Autodesk Inventor part; units mm, degrees
ref_plane "YZ Plane" through (0, 0, 0) normal (1, 0, 0) x (0, 1, 0)
ref_plane "XZ Plane" through (0, 0, 0) normal (0, 1, 0) x (-1, 0, 0)
ref_plane "XY Plane" through (0, 0, 0) normal (0, 0, 1) x (1, 0, 0)
sketch "Sketch1" plane through (0, 0, 0) normal (0, 1, 0) x (-1, 0, 0)
  line L0 (900, 40) -> (-900, 40)
  line L1 (-900, 40) -> (-900, -40)
  line L2 (-900, -40) -> (900, -40)
  line L3 (900, -40) -> (900, 40)
  line L4 (900, 40) -> (-900, -40) construction
  line L5 (674.96, 40) -> (721.148, -40)
  line L6 (0, 40) -> (0, -40) construction
  line L7 (-674.96, 40) -> (-721.148, -40)
  point P0 (0, 0)
  point P1 (0, 0)
  dimension "d0" = 80
  dimension "d1" = 1800
  dimension "d3" = 120
  dimension "d6" = 674.96
  dimension "d7" = 120
  dimension "d8" = 674.96
extrude "Plate1" add sketch "Sketch1" along normal mid plane 3 contours L5 L2 L7 L0
sketch "Sketch2" plane through (0, -1.5, 0) normal (0, -1, 0) x (1, 0, 0)
  line L0 (-1.6, 40) -> (1.6, 40)
  line L1 (1.6, 40) -> (1.6, -1)
  line L2 (1.6, -1) -> (-1.6, -1)
  line L3 (-1.6, -1) -> (-1.6, 40)
  line L4 (-674.96, 40) -> (674.96, 40)
  point P0 (0, 0)
  point P1 (0, 40)
  dimension "d9" = 3.2
  dimension "d10" = 41
extrude "Extrusion1" cut sketch "Sketch2" against normal through all
pattern_linear "Rectangular Pattern1" count 5 spacing 240 along (1, 0, 0) of "Extrusion1" first direction both ways yes
equation "\"d7\" = d3"
equation "\"d8\" = d6"
equation "\"d2\" = Thickness"
equation "\"BendReliefWidth\" = Thickness"
equation "\"BendReliefDepth\" = 0.5 * Thickness"
equation "\"CornerReliefSize\" = 4 * Thickness"
equation "\"MinimumRemnant\" = 2 * Thickness"
equation "\"TransitionRadius\" = BendRadius"
equation "\"JacobiRadiusSize\" = BendRadius"
equation "\"GapSize\" = Thickness"
properties part number "MSC 203 GRID" material "Stainless Steel"
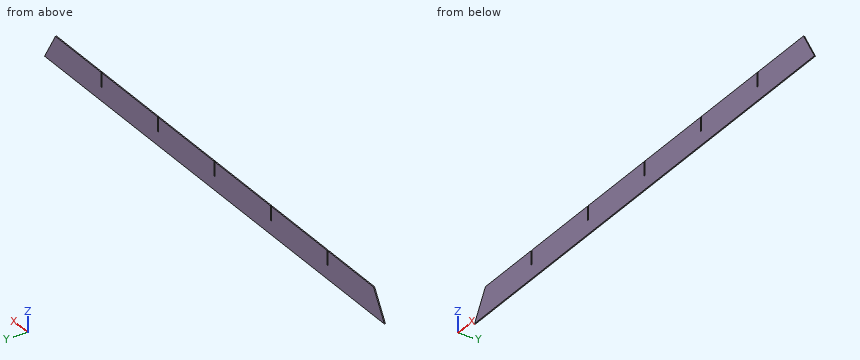
Check sheet for the modelled part. Datum: model origin and axes. Units: mm. Round coordinates to 2 decimals unless told otherwise and drop trailing zeros. Write each loop counter-clockwise with the first axis right and the second up, starting at its lowest first coordinate (ties: lowest second). Pieces come first, ordered by that corner, then holes. Notation, with made-up numbers: (-30.75, -2.75) -> (-20.75, -2.75) arc R20 cw to (-20.75, 34.25) -> close; hole circle Ø11 at (49.25, -6). An arc over 180 degrees is marked (long way). One line per question, with ' | ' between items. Start each with the question number.
1. Sectioned sample at B-B, the plane z = 25.5. Record the cut outline in (x, y), then the cut area to 3 significant figures.
2. Sectioned sample at A-A, the plane y = 0.3. Record the cut outline in (x, z), then the cut area to 3 significant figures.
3. Depth check by flat-ended pin: pin 1 (0.9 mm diameter, centred on x = 0, y = 0, fed in from +Z); pin 2 (1.5 mm diameter, centred on y = 0.5, z = 25.5, fed in from +X); pin 3 (0.9 mm diameter, centred on y = 0, z = 23.5, fed in from +X). Enter the tip coordinate at first touch or a pass-through.
4. Scan lines: line 1 along X through (y, z) = (0.1, 20); line 2 along X through (y, z) = (-1.3, 24); line 3 along X through (y, z) = (0.35, -32). Record each from-to range of solid material in increasing order. Write a range as from..to.
Taken from the geometry:
1) outline: (-683.33, -1.5) -> (-481.6, -1.5) -> (-481.6, 1.5) -> (-683.33, 1.5) -> close; (-478.4, -1.5) -> (-241.6, -1.5) -> (-241.6, 1.5) -> (-478.4, 1.5) -> close; (-238.4, -1.5) -> (-1.6, -1.5) -> (-1.6, 1.5) -> (-238.4, 1.5) -> close; (1.6, -1.5) -> (238.4, -1.5) -> (238.4, 1.5) -> (1.6, 1.5) -> close; (241.6, -1.5) -> (478.4, -1.5) -> (478.4, 1.5) -> (241.6, 1.5) -> close; (481.6, -1.5) -> (683.33, -1.5) -> (683.33, 1.5) -> (481.6, 1.5) -> close | area: 4,050 mm^2
2) outline: (-721.15, -40) -> (721.15, -40) -> (674.96, 40) -> (481.6, 40) -> (481.6, -1) -> (478.4, -1) -> (478.4, 40) -> (241.6, 40) -> (241.6, -1) -> (238.4, -1) -> (238.4, 40) -> (1.6, 40) -> (1.6, -1) -> (-1.6, -1) -> (-1.6, 40) -> (-238.4, 40) -> (-238.4, -1) -> (-241.6, -1) -> (-241.6, 40) -> (-478.4, 40) -> (-478.4, -1) -> (-481.6, -1) -> (-481.6, 40) -> (-674.96, 40) -> close | area: 111,000 mm^2
3) pin 1: stops at z = -1 | pin 2: stops at x = 683.76 | pin 3: stops at x = 684.75
4) line 1: x = -686.51..-481.6, -478.4..-241.6, -238.4..-1.6, 1.6..238.4, 241.6..478.4, 481.6..686.51 | line 2: x = -684.2..-481.6, -478.4..-241.6, -238.4..-1.6, 1.6..238.4, 241.6..478.4, 481.6..684.2 | line 3: x = -716.53..716.53
